```python
from build123d import *

# Parameters (mm, degrees)
BOSS_EXTRUDE1_DEPTH = 19.05
SKETCH4_R           = 22.5
CUT_EXTRUDE1_DEPTH  = 17.05
FILLET1_R           = 1


with BuildPart() as part:
    # Sketch1 → Boss-Extrude1 (new body)
    with BuildSketch(Plane.XY):
        with BuildLine():
            Line((14.641905013, 96.116783887), (29.641905013, 96.116783887))
            Line((29.641905013, 96.116783887), (29.641905013, 55.878392582))
            ThreePointArc((29.641905013, 55.878392582), (94.077954609, 36.943795037), (29.641905013, 18.009197492))
            Line((29.641905013, 18.009197492), (29.641905013, 6.116783887))
            Line((29.641905013, 6.116783887), (14.641905013, 6.116783887))
            Line((14.641905013, 6.116783887), (14.641905013, 96.116783887))
        make_face()
    extrude(amount=BOSS_EXTRUDE1_DEPTH)

    # Sketch4 → Cut-Extrude1 (cut)
    with BuildSketch(Plane.XY.offset(19.05)):
        with BuildLine():
            Line((28.486331549, 21.619208615), (28.486331549, 7.023321428))
            Line((28.486331549, 7.023321428), (15.986331549, 7.023321428))
            Line((15.986331549, 7.023321428), (15.986331549, 94.523321428))
            Line((15.986331549, 94.523321428), (28.486331549, 94.523321428))
            Line((28.486331549, 94.523321428), (28.486331549, 51.962640383))
            ThreePointArc((28.486331549, 51.962640383), (92.383993766, 36.790924499), (28.486331549, 21.619208615))
        make_face()
        with Locations((58.633993766, 36.790924499)):
            Circle(SKETCH4_R, mode=Mode.SUBTRACT)
    extrude(amount=-CUT_EXTRUDE1_DEPTH, mode=Mode.SUBTRACT)

    # Fillet1
    fillet1_edges = [part.edges().sort_by_distance(p)[0] for p in [
        (22.236331549, 7.023321428, 2),
        (28.486331549, 7.023321428, 10.525),
        (15.986331549, 50.773321428, 2),
        (15.986331549, 7.023321428, 10.525),
        (15.986331549, 94.523321428, 10.525),
        (28.486331549, 73.242980906, 2),
        (28.486331549, 94.523321428, 10.525),
        (92.383993766, 36.790924499, 2),
        (28.486331549, 51.962640383, 10.525),
        (28.486331549, 14.321265022, 2),
        (28.486331549, 21.619208615, 10.525),
    ]]
    fillet(fillet1_edges, radius=FILLET1_R)


solid = part.part
```
Work out the finished part from the listing and answer in its coordinate system (mm). A direction names the side the tool comes from. Round coordinates to 2 decimals unless told otherwise and drop trailing zeros. Write each loop counter-clockwise with the first axis right and the second up, starting at its lowest first coordinate (ties: lowest second). Pieces come first, ordered by that corner, then holes. Notation, with made-up numbers: (-1.5, 12) - (40.5, 12) arc R32 ccw to (40.5, 42) - close; hole circle Ø7 at (80.5, 71). An arc over 180 degrees is marked (long way). Return JSON: item names as keys, results as strings. Group by question number.
Q1. The part is cut by section C-C on y = 81.5. Write down the section's boundary in (x, z), then the cut area to 3 significant figures.
Q2. Find the intervals of material crossed by L1, parallel to X at y = 73, z = 10; L2, parallel to Y at x = 57, z = 10.75; L3, parallel to X at y = 43, z = 16, in increasing order.
Q3. The mould has two halves that part along Y. Classify faces 4 (the flat face through (59, 37, 19.05)), 5 (the cylindrical face through (80.095, 43.549, 10.644)), 6 (the flat face through (22, 6.117, 9)): released by +Y, released by -Y, zero draft, split by the parting line, or undercut.
Q4. For faces 1 (the flat face through (29.642, 76, 9)), 2 (the flat face through (28.486, 13, 11)), 3 (the flat face through (22, 96.117, 9)), determine the directions among +Z, -Z, +X, -X, +Y, -Y from which every point of the face is accessible in a straight line to the end or side of a thin tool.
Q5. Each of these flat-tipped pins is pushed along its axis until it touches: pin 1 Ø1.5 at (x, z) = (59.5, 6) entering from +Y; pin 2 Ø6 at (x, z) = (84, 9) entering from +Y; pin 3 Ø9.5 at (y, z) = (68.5, 7) entering from +X. Where does it stop, or does it pass through?
Q6. The part is cut by section A-A on z = 17.5. Write down the section's boundary in (x, y).
Q7. The part is cut by section B-B on x = 24. Write down the section's boundary in (y, z).
Solved:
{
 "1": {"outline": "(14.64, 0) - (29.64, 0) - (29.64, 19.05) - (28.49, 19.05) - (28.49, 3) arc R1 cw to (27.49, 2) - (16.99, 2) arc R1 cw to (15.99, 3) - (15.99, 19.05) - (14.64, 19.05) - close", "area": "73.1 mm²"},
 "2": {"L1": "14.64 to 15.99, 28.49 to 29.64", "L2": "2.01 to 3.08, 14.35 to 59.23, 70.5 to 71.88", "L3": "14.64 to 15.99, 37.01 to 80.26, 91.81 to 93.55"},
 "3": {"face 4": "zero draft", "face 5": "undercut", "face 6": "released by -Y"},
 "4": {"face 1": "+Z, -Z, +Y", "face 2": "+Z", "face 3": "+Z, -Z, +X, -X, +Y"},
 "5": {"pin 1": "y = 71.94", "pin 2": "y = 64.23", "pin 3": "x = 81.58"},
 "6": {"outline": "(14.64, 6.12) - (29.64, 6.12) - (29.64, 18.01) arc R35 ccw (long way) to (29.64, 55.88) - (29.64, 96.12) - (14.64, 96.12) - close; circle Ø45 at (58.63, 36.79); hole (15.99, 8.02) arc R1 ccw to (16.99, 7.02) - (27.49, 7.02) arc R1 ccw to (28.49, 8.02) - (28.49, 17.87) arc R1 cw to (30.33, 18.42) arc R33.75 ccw (long way) to (30.33, 55.17) arc R1 cw to (28.49, 55.71) - (28.49, 93.52) arc R1 ccw to (27.49, 94.52) - (16.99, 94.52) arc R1 ccw to (15.99, 93.52) - close"},
 "7": {"outline": "(6.12, 0) - (96.12, 0) - (96.12, 19.05) - (94.52, 19.05) - (94.52, 2) - (8.02, 2) arc R1 cw to (7.02, 3) - (7.02, 19.05) - (6.12, 19.05) - close"}
}
